```python
from build123d import *

# Parameters (mm, degrees)
F0_W     = 6.35
F0_H     = 6.35
F1_DEPTH = 6.35
F2_R     = 3.175
F3_DEPTH = 3.96875
F4_R     = 2.38125
F5_DEPTH = 8.73125
F6_R     = 1.7272
F7_DEPTH = 6.35
F8_SIZE  = 0.79375


with BuildPart() as f1:
    # F0 (on Top) → F1 (new body)
    with BuildSketch(Plane.XY):
        Rectangle(F0_W, F0_H)
    extrude(amount=F1_DEPTH)

    # F2 (on Front) → F3 (join, symmetric)
    with BuildSketch(Plane.XZ):
        with Locations((0, 3.175)):
            Circle(F2_R)
    extrude(amount=F3_DEPTH, both=True)

    # F4 (on Front) → F5 (join, symmetric)
    with BuildSketch(Plane.XZ):
        with Locations((0, 3.175)):
            Circle(F4_R)
    extrude(amount=F5_DEPTH, both=True)

    # F6 (on face) → F7 (cut, through all)
    with BuildSketch(Plane(origin=(0, 0, 0), x_dir=(1, 0, 0), z_dir=(0, 0, -1))):
        Circle(F6_R)
    extrude(amount=-F7_DEPTH, mode=Mode.SUBTRACT)

    # F8
    f8_edges = [f1.edges().sort_by_distance(p)[0] for p in [
        (-2.38125, -8.73125, 3.175),
        (-2.38125, 8.73125, 3.175),
    ]]
    chamfer(f8_edges, length=F8_SIZE)


solid = f1.part
```
Model file for the job. Use its own axes, mm. A direction names the side the tool comes from. Give positions to 0.01 mm unless a question says otherwise; leave off trailing zeros. Write each loop counter-clockwise with the first axis right and the second up, starting at its lowest first coordinate (ties: lowest second). Pieces come first, ordered by that corner, then holes. Notation, with made-up numbers: (34, 59) -> (78, 59) arc R12 ccw to (78, 79) -> close; hole circle Ø10 at (47.25, 7.25). An arc over 180 degrees is marked (long way). Use CSV: the item, a comma, the result in double quotes. Start each with the question number.
1) Cut at A-A on y = 0. List the corners of the cut face in (x, z) (3 decimals).
2) Cut at B-B on z = 0.5. List the corners of the cut face in (x, y) (3 decimals).
3) Pin check, flat tip, straight feed: P1, Ø1, axis at x = 2, z = 5, coming from the +Y side. Stop position of the tip, or through.
4) Cut at C-C on y = 5. List the corners of the cut face in (x, z) (1 decimal), plus the area to 3 significant figures.
5) Drill centre lines: L1, parallel to X at y = 0, z = 2 (3 decimals); L2, parallel to Y at x = 0, z = 2; L3, parallel to Y at x = -2.5, z = 2.25. Where is each one in solid material? Low to high.
6) Tool access for faces 1 (the flat face through (-3, -3.175, 1)), 2 (the flat face through (-3, 3.175, 1)), 3 (the flat face through (0, -3.969, 6)): list every direction of +Z, -Z, +X, -X, +Y, -Y with a clear straight run to the whole face (end or side of a thin tool).
Final values:
1,outline,"(-3.175, 0) -> (-1.727, 0) -> (-1.727, 6.35) -> (-3.175, 6.35) -> close; (1.727, 0) -> (3.175, 0) -> (3.175, 6.35) -> (1.727, 6.35) -> close"
2,outline,"(-3.175, -3.175) -> (-1.71, -3.175) -> (-1.71, -3.969) -> (1.71, -3.969) -> (1.71, -3.175) -> (3.175, -3.175) -> (3.175, 3.175) -> (1.71, 3.175) -> (1.71, 3.969) -> (-1.71, 3.969) -> (-1.71, 3.175) -> (-3.175, 3.175) -> close; hole circle Ø3.454 at (0, 0)"
3,P1,"stops at y = 8.11"
4,outline,"circle Ø4.8 at (0, 3.2)"
4,area,"17.8 mm2"
5,L1,"x = -3.175 to -1.727, 1.727 to 3.175"
5,L2,"y = -8.73 to -1.73, 1.73 to 8.73"
5,L3,"y = -3.97 to 3.97"
6,face 1,"-Z, -X, -Y"
6,face 2,"-Z, -X, +Y"
6,face 3,"-Y"
